The model under review builds one solid part; all positions refer to its coordinate system, in mm. Face numbers are marked on the shaded views. A direction names the side the tool comes from. Round coordinates to 2 decimals unless told otherwise and drop trailing zeros. Order: outer loops, then holes, each group sorted by start corner. A loop starts at its lowest first (then second) coordinate and runs counter-clockwise, first axis right, second up. Notation, with made-up numbers: M 68.25,6 L 107.25,6 A32 ccw 107.25,33 Z; hole C 86,-3 d3. An arc over 180 degrees is marked long. Answer as a JSON object with one key per item and string values. Group by question number.
1) Consider section A-A, the plane z = 15. Write out the cut boundary in (x, y).
2) Consider section C-C, the plane y = 56. Write out the cut boundary in (x, z), then the cut area to 3 significant figures.
3) Insertion check: pin 1 Ø6 at (y, z) = (-78.5, 5.5) entering from +X; pin 2 Ø12 at (x, z) = (2, -9) entering from -Y; pin 3 Ø8 at (x, z) = (27, 7) entering from -Y; pin 4 Ø19.5 at (x, y) = (70, -76.5) entering from +Z. Each pin has a flat end and moves straight along its axis. Give the tip position at first contact, or say it passes through.
4) The part is to be moulded in two halves that separate along X. For the marked faces 4, 5 and 6, say which applies: +X half, -X half, draft (parallel to the pull), parting line (faces both ways), or undercut.
5) To check wall thickness, follow line 1 (Y direction, x = 70, z = 8.75); line 2 (Y direction, x = 70, z = -7.5); line 3 (Z direction, x = -62, y = -61). State the ranges of each line that lie inside material, in increasing order.
6) For the marked faces 1, 2 and 3, list the 3-axis set-ups (+Z, -Z, +X, -X, +Y, -Y) from which the entire face can be reached by the end or side of a thin tool; tool diameter is ignored.
7) Consider section D-D, the plane z = -40. Write out the cut boundary in (x, y), then the cut area to 3 significant figures.
8) Consider section B-B, the plane x = -62.5. Write out the cut boundary in (y, z).
```python
from build123d import *

# Parameters (mm, degrees)
SKETCH1_W                               = 200
SKETCH1_H                               = 213
BOSS_EXTRUDE1_DEPTH                     = 25
BOSS_EXTRUDE2_DEPTH                     = 10
BOSS_EXTRUDE3_DEPTH                     = 70
CUT_EXTRUDE1_DEPTH                      = 20
BOSS_EXTRUDE5_DEPTH                     = 10
BOSS_EXTRUDE5_DEPTH_BACK                = 120
SKETCH5_R                               = 35
BOSS_EXTRUDE6_DEPTH                     = 10
BOSS_EXTRUDE6_DEPTH_BACK                = 120
SKETCH6_R                               = 41.5
CUT_EXTRUDE2_REACH                      = 274.509
SKETCH7_R                               = 20.5
CUT_EXTRUDE3_REACH                      = 209.134
SKETCH8_R                               = 20.5
CBORE_FOR_M8_HEX_HEAD_BOLT1_D           = 15
CBORE_FOR_M8_HEX_HEAD_BOLT1_CBORE_D     = 30
CBORE_FOR_M8_HEX_HEAD_BOLT1_CBORE_DEPTH = 10
CHAMFER1_SIZE                           = 2
FILLET1_R                               = 10


with BuildPart() as part:
    # Sketch1 → Boss-Extrude1 (new body)
    with BuildSketch(Plane.XY):
        Rectangle(SKETCH1_W, SKETCH1_H)
    extrude(amount=BOSS_EXTRUDE1_DEPTH)

    # Sketch2 → Boss-Extrude2 (add)
    with BuildSketch(Plane.XY):
        with BuildLine():
            Line((100, -46.5), (55, -46.5))
            ThreePointArc((55, -46.5), (44.393398282, -50.893398282), (40, -61.5))
            Line((40, -61.5), (40, -106.5))
            Line((40, -106.5), (100, -106.5))
            Line((100, -106.5), (100, -46.5))
        make_face()
    extrude(amount=-BOSS_EXTRUDE2_DEPTH)

    # Sketch3 → Boss-Extrude3 (add)
    with BuildSketch(Plane(origin=(0, 0, 0), x_dir=(-1, 0, 0), z_dir=(0, 0, -1))):
        with BuildLine():
            Line((-100, 63.5), (-20, 63.5))
            ThreePointArc((-20, 63.5), (6.360389693, -0.139610307), (70, -26.5))
            Line((70, -26.5), (70, -106.5))
            Line((70, -106.5), (55, -106.5))
            Line((55, -106.5), (55, -41.5))
            ThreePointArc((55, -41.5), (-4.246212025, -10.746212025), (-35, 48.5))
            Line((-35, 48.5), (-100, 48.5))
            Line((-100, 48.5), (-100, 63.5))
        make_face()
    extrude(amount=BOSS_EXTRUDE3_DEPTH)

    # Sketch4 → Cut-Extrude1 (cut)
    with BuildSketch(Plane(origin=(0, 0, 0), x_dir=(-1, 0, 0), z_dir=(0, 0, -1))):
        with BuildLine():
            Line((-42.323661941, 39.5), (-91, 39.5))
            Line((-91, 39.5), (-91, -37.5))
            Line((-91, -37.5), (-55, -37.5))
            ThreePointArc((-55, -37.5), (-38.029437252, -44.529437252), (-31, -61.5))
            Line((-31, -61.5), (-31, -97.5))
            Line((-31, -97.5), (46, -97.5))
            Line((46, -97.5), (46, -48.823661941))
            ThreePointArc((46, -48.823661941), (-10.610173055, -17.110173055), (-42.323661941, 39.5))
        make_face()
    extrude(amount=-CUT_EXTRUDE1_DEPTH, mode=Mode.SUBTRACT)

    # Sketch5 → Boss-Extrude5 (add, two sides: drawn at the far end of the back side and taken through both)
    with BuildSketch(Plane(origin=(100, 0, 0), x_dir=(0, 0, -1), z_dir=(1, 0, 0)).offset(-BOSS_EXTRUDE5_DEPTH_BACK)):
        with Locations((70, 56)):
            Circle(SKETCH5_R)
    extrude(amount=BOSS_EXTRUDE5_DEPTH + BOSS_EXTRUDE5_DEPTH_BACK)

    # Sketch6 → Boss-Extrude6 (add, two sides: drawn at the far end of the back side and taken through both)
    with BuildSketch(Plane.XZ.offset(106.5).offset(-BOSS_EXTRUDE6_DEPTH_BACK)):
        with Locations(Location((-62.5, -70, 0), (0, 0, 270))):
            Circle(SKETCH6_R)
    extrude(amount=BOSS_EXTRUDE6_DEPTH + BOSS_EXTRUDE6_DEPTH_BACK)

    # Sketch7 → Cut-Extrude2 (cut, up to next)
    with BuildSketch(Plane.XZ.offset(116.5), mode=Mode.PRIVATE) as cut_extrude2_sk1:
        with Locations(Location((-62.5, -70, 0), (0, 0, 270))):
            Circle(SKETCH7_R)
    cut_extrude2_tool1 = extrude(cut_extrude2_sk1.sketch, amount=-CUT_EXTRUDE2_REACH, mode=Mode.PRIVATE) & part.part
    add(cut_extrude2_tool1.solids().sort_by_distance((-62.5, -116.5, -70))[0], mode=Mode.SUBTRACT)

    # Sketch8 → Cut-Extrude3 (cut, up to next)
    with BuildSketch(Plane.ZY.offset(20), mode=Mode.PRIVATE) as cut_extrude3_sk1:
        with Locations((-70, 56)):
            Circle(SKETCH8_R)
    cut_extrude3_tool1 = extrude(cut_extrude3_sk1.sketch, amount=-CUT_EXTRUDE3_REACH, mode=Mode.PRIVATE) & part.part
    add(cut_extrude3_tool1.solids().sort_by_distance((-20, 56, -70))[0], mode=Mode.SUBTRACT)

    # CBORE for M8 Hex Head Bolt1 (through all)
    with Locations(Plane(origin=(70, -76.5, -10), x_dir=(-1, 0, 0), z_dir=(0, 0, -1))):
        with Locations((0, 0)):
            CounterBoreHole(CBORE_FOR_M8_HEX_HEAD_BOLT1_D / 2, CBORE_FOR_M8_HEX_HEAD_BOLT1_CBORE_D / 2, CBORE_FOR_M8_HEX_HEAD_BOLT1_CBORE_DEPTH)

    # Chamfer1
    chamfer1_edges = [part.edges().sort_by_distance(p)[0] for p in [
        (-62.5, -116.5, -49.5),
        (-62.5, 13.5, -49.5),
        (110, 56, -90.5),
        (-20, 56, -90.5),
    ]]
    chamfer(chamfer1_edges, length=CHAMFER1_SIZE)

    # Fillet1
    fillet1_edges = [part.edges().sort_by_distance(p)[0] for p in [
        (42.323661941, 39.5, 10),
        (-46, -48.823661941, 10),
        (-46, -97.5, 10),
        (31, -97.5, 10),
        (91, -37.5, 10),
        (91, 39.5, 10),
        (100, -106.5, 7.5),
        (-100, -106.5, 12.5),
        (-100, 106.5, 12.5),
        (100, 106.5, 12.5),
    ]]
    fillet(fillet1_edges, radius=FILLET1_R)


solid = part.part
```
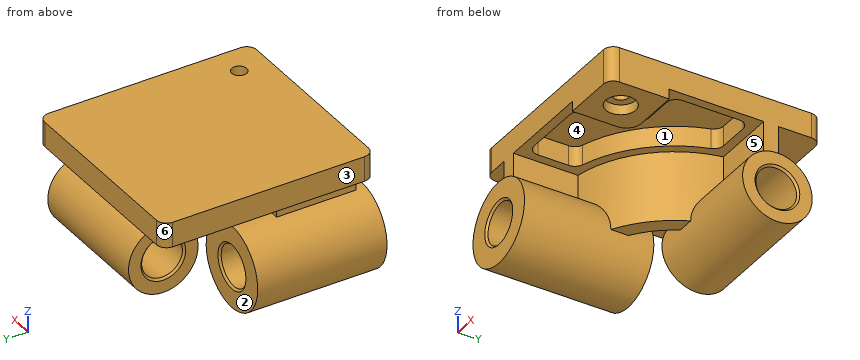
Results list:
{
 "1": {"outline": "M -100,-96.5 A10 ccw -90,-106.5 L 90,-106.5 A10 ccw 100,-96.5 L 100,96.5 A10 ccw 90,106.5 L -90,106.5 A10 ccw -100,96.5 Z; hole M -46,-87.5 A10 ccw -36,-97.5 L 21,-97.5 A10 ccw 31,-87.5 L 31,-61.5 A24 cw 55,-37.5 L 81,-37.5 A10 ccw 91,-27.5 L 91,29.5 A10 ccw 81,39.5 L 49.95,39.5 A10 ccw 40.39,32.43 A119.58 cw -38.93,-46.89 A10 ccw -46,-56.45 Z; hole C 70,-76.5 d15"},
 "2": {"outline": "M -100,0 L 19.69,0 L 19.69,-35 L -20,-35 L -20,-47.5 L -18,-49.5 L 108,-49.5 L 110,-47.5 L 110,-35 L 100,-35 L 100,25 L -100,25 Z; M -20,-105 L 110,-105 L 110,-92.5 L 108,-90.5 L -18,-90.5 L -20,-92.5 Z", "area": "11,600 mm^2"},
 "3": {"pin 1": "x = 100", "pin 2": "y = -18.2", "pin 3": "y = -106.5", "pin 4": "z = 25"},
 "4": {"face 4": "undercut", "face 5": "draft", "face 6": "-X half"},
 "5": {"line 1": "-106.5 to -84, -69 to -37.5, 39.5 to 106.5", "line 2": "-106.5 to -91.5, -61.5 to -46.5, 48.5 to 63.5", "line 3": "-111.5 to -90.49, -49.51 to 25"},
 "6": {"face 1": "none", "face 2": "-Z, -X, +Y", "face 3": "+Z, -X, +Y, -Y"},
 "7": {"outline": "M -91.17,-116.5 L -33.83,-116.5 L -33.83,-35.6 A110.58 ccw 32.63,37.97 L 110,37.97 L 110,74.03 L -20,74.03 L -20,37.97 L 16.3,37.97 A90 cw -33.83,-18.91 L -33.83,13.5 L -91.17,13.5 Z", "area": "13,500 mm^2"},
 "8": {"outline": "M -116.5,-111.5 L 13.5,-111.5 L 13.5,-92.5 L 11.5,-90.5 L -114.5,-90.5 L -116.5,-92.5 Z; M -116.5,-47.5 L -114.5,-49.5 L 11.5,-49.5 L 13.5,-47.5 L 13.5,-28.5 L -26.19,-28.5 L -26.19,0 L 106.5,0 L 106.5,25 L -106.5,25 L -106.5,-28.5 L -116.5,-28.5 Z"}
}
